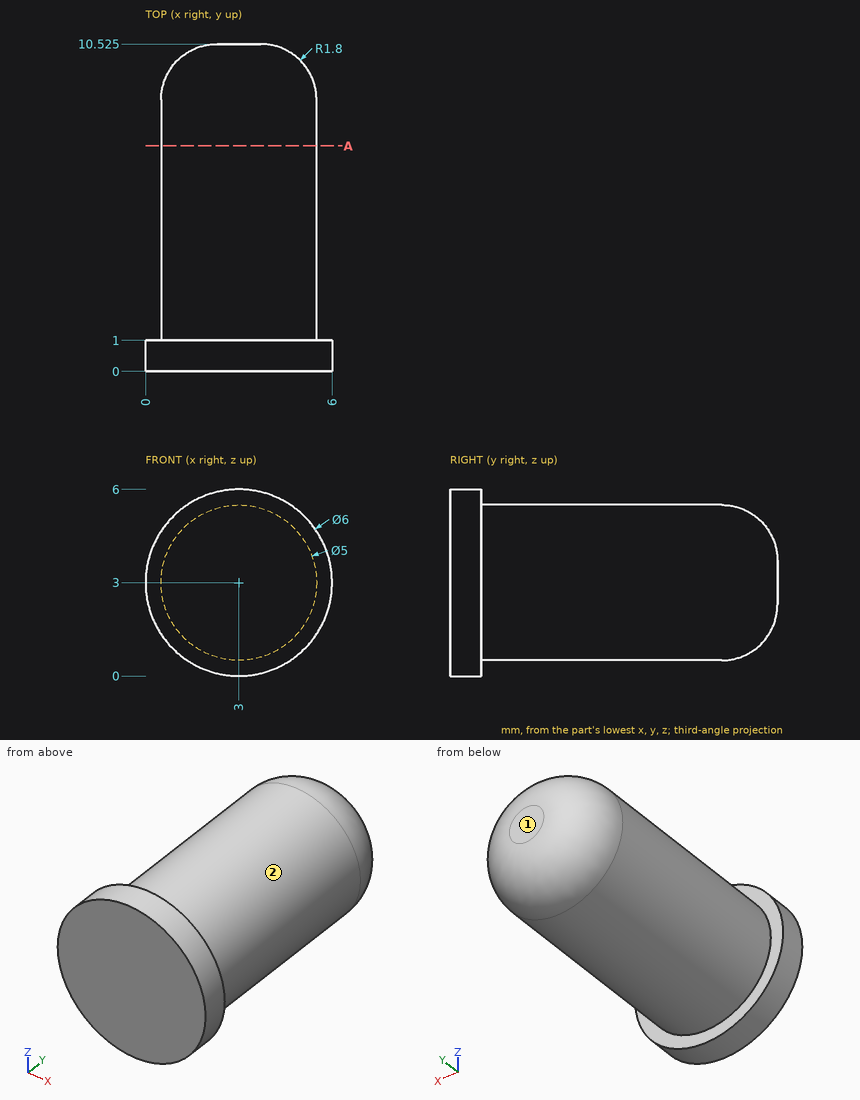
Design review of the part shown in the three views and the two pictorial views. Dimensions are in mm from the part's minimum x, y and z. A direction names the side the tool comes from. Coordinates: 2 decimals unless noted, no trailing zeros. Order: outer loops, then holes, each group sorted by start corner. A loop starts at its lowest first (then second) coordinate and runs counter-clockwise, first axis right, second up.
Item 1: For pin 1 Ø1.5 at (x, y) = (4, 7.5) entering from +Z; pin 2 Ø1.5 at (y, z) = (7.5, 4) entering from -X, all flat-tipped, find the tip position at first contact; note any pin that passes through.
Item 2: For the marked faces 1 and 2, list the 3-axis set-ups (+Z, -Z, +X, -X, +Y, -Y) from which the entire face can be reached by the end or side of a thin tool; tool diameter is ignored.
Item 3: Take a section at A-A, the plane y = 7.25. Write out the cut boundary in (x, z), then the cut area to 3 significant figures.
Item 4: For line 1 (Y direction, x = 0.5, z = 4.05); line 2 (Z direction, x = 1.6, y = 1.25); line 3 (Z direction, x = 3.7, y = 3.5), list the stretches that pass through material, from the lowest coordinate up.
The answers:
1. pin 1: stops at z = 5.49
1. pin 2: stops at x = 0.51
2. face 1: +Z, -Z, +X, -X, +Y
2. face 2: +Y
3. outline: circle Ø5 at (3, 3)
3. area: 19.6 mm2
4. line 1: y = 0 to 1
4. line 2: z = 0.93 to 5.07
4. line 3: z = 0.6 to 5.4
